from build123d import *

# Parameters (mm, degrees)
F1_DEPTH = 12.7
F2_W     = 114.3
F2_H     = 184.15
F3_DEPTH = 12.7
F4_R     = 25.4
F5_D     = 14.224
F6_D     = 19.812
F7_D     = 7.112
F8_R     = 25.4


with BuildPart() as f1:
    # F0 (on Front) → F1 (new body)
    with BuildSketch(Plane.XZ):
        Polygon((-400.558, 0), (0, 0), (0, 457.2), align=None)
    extrude(amount=F1_DEPTH)

    # F2 (on face) → F3 (cut, through all)
    with BuildSketch(Plane.XZ.offset(12.7)):
        with Locations((-69.85, 111.125)):
            Rectangle(F2_W, F2_H)
        Polygon((-205.64757, 203.2), (-366.983431, 19.05), (-140.716, 19.05), (-140.716, 203.2), align=None)
        Polygon((-12.7, 355.6), (-72.128237, 355.6), (-194.520959, 215.9), (-12.7, 215.9), align=None)
    extrude(amount=-F3_DEPTH, mode=Mode.SUBTRACT)

    # F4
    f4_edges = [f1.edges().sort_by_distance(p)[0] for p in [
        (-205.64757, -6.35, 203.2),
        (-140.716, -6.35, 203.2),
        (-127, -6.35, 203.2),
        (-12.7, -6.35, 203.2),
        (-12.7, -6.35, 355.6),
        (-72.128237, -6.35, 355.6),
        (-366.983431, -6.35, 19.05),
        (-140.716, -6.35, 19.05),
        (-127, -6.35, 19.05),
        (-12.7, -6.35, 19.05),
        (-194.520959, -6.35, 215.9),
        (-12.7, -6.35, 215.9),
    ]]
    fillet(f4_edges, radius=F4_R)

    # F5 (through all)
    with Locations(Plane.XZ.offset(12.7)):
        with Locations((-349.758, 25.4)):
            Hole(F5_D / 2)

    # F6 (through all)
    with Locations(Plane.XZ.offset(12.7)):
        with Locations((-25.4, 390.398)):
            Hole(F6_D / 2)

    # F7 (through all)
    with Locations(Plane.XZ.offset(12.7)):
        with Locations((-228.6, 9.525), (-133.35, 9.525), (-133.35, 47.752), (-6.35, 47.752), (-12.7, 9.525)):
            Hole(F7_D / 2)

    # F8
    f8_edges = [f1.edges().sort_by_distance(p)[0] for p in [
        (0, -6.35, 457.2),
        (-400.558, -6.35, 0),
    ]]
    fillet(f8_edges, radius=F8_R)


solid = f1.part
Design review of the part built by this model. Coordinates are the model's own, in mm. A direction names the side the tool comes from. Round coordinates to 2 decimals unless told otherwise and drop trailing zeros. Write each loop counter-clockwise with the first axis right and the second up, starting at its lowest first coordinate (ties: lowest second). Pieces come first, ordered by that corner, then holes. Notation, with made-up numbers: M -32.75,77 L -26.75,77 A12 ccw -26.75,86 Z; hole C 4.25,-18.5 d9. An arc over 180 degrees is marked long. One line per item, written item: value. Start each with the question number.
1. Draft analysis for pull direction X (two halves, no side actions). For faces 1 (the face through (0, -6, 192)), 2 (the face through (-20.34, -6.26, 223.14)), 3 (the face through (-131, 0, 147)), state which applies: pulls with the +X half, pulls with the -X half, needs draft (parallel to the pull), parting line crosses it, or undercut.
2. Clearance check with flat-ended pins moving along their axes: P1, Ø5, axis at x = -157.5, y = -7, coming from the +Z side; P2, Ø6.5, axis at x = -265, y = -5.5, coming from the +Z side; P3, Ø6.5, axis at x = -70.5, y = -8.5, coming from the +Z side. State where each tip first meets the part, or that it passes through.
3. Take a section at D-D on y = -4.5. State how many separate pieces and enclosed holes the cut face has, then the cut area to 3 significant figures.
4. To check wall thickness, follow probe 1 along X at (y, z) = (-3.25, 33); probe 2 along Z at (x, y) = (-228.6, -7.25); probe 3 along Z at (x, y) = (-25, -5). State the ranges of each line that lie inside material, in increasing order. Write a range as from..to.
5. Take a section at A-A on x = -25.4. State the section outline as (y, z) points.
6. For faces 4 (the face through (-131, -12.7, 147)), 5 (the face through (-20.34, -6.26, 348.36)), list the 3-axis set-ups (+Z, -Z, +X, -X, +Y, -Y) from which the entire face can be reached by the end or side of a thin tool; tool diameter is ignored.
7. Take a section at C-C on z = 25.4. State the section outline as (x, y) points, then the cut area to 3 significant figures.
8. Take a section at B-B on z = 385. State the section outline as (x, y) points.
Computed:
1. face 1: pulls with the +X half
1. face 2: undercut
1. face 3: needs draft
2. P1: stops at z = 280.28
2. P2: stops at z = 158.44
2. P3: stops at z = 380.44
3. separate pieces: 1
3. enclosed holes: 10
3. area: 27,100 mm²
4. probe 1: x = -368.77..-333.63, -143.44..-124.27, -15.43..0
4. probe 2: z = 0..5.97, 13.08..19.05, 177..196.27
4. probe 3: z = 0..22.69, 199.56..219.54, 351.96..380.5, 400.3..415.06
5. outline: M -12.7,0 L 0,0 L 0,22.45 L -12.7,22.45 Z; M -12.7,199.8 L 0,199.8 L 0,219.3 L -12.7,219.3 Z; M -12.7,352.2 L 0,352.2 L 0,380.49 L -12.7,380.49 Z; M -12.7,400.3 L 0,400.3 L 0,415.06 L -12.7,415.06 Z
6. face 4: +Z, -Z, +X, -X, -Y
6. face 5: +Y, -Y
7. outline: M -369.94,-12.7 L -356.87,-12.7 L -356.87,0 L -369.94,0 Z; M -342.65,-12.7 L -327.76,-12.7 L -327.76,0 L -342.65,0 Z; M -149.32,-12.7 L -118.4,-12.7 L -118.4,0 L -149.32,0 Z; M -21.3,-12.7 L 0,-12.7 L 0,0 L -21.3,0 Z
7. area: 1,020 mm²
8. outline: M -63.26,-12.7 L -33.71,-12.7 L -33.71,0 L -63.26,0 Z; M -17.09,-12.7 L 0,-12.7 L 0,0 L -17.09,0 Z
